```python
from build123d import *

# Parameters (mm, degrees)
SALIENTE_EXTRUIR1_DEPTH = 1.5


with BuildPart() as part:
    # Croquis1 → Saliente-Extruir1 (new, symmetric)
    with BuildSketch(Plane.XY):
        Polygon((484.855720511, 82.973038085), (491.215178715, 82.973038085), (501.205555648, 82.973038085), (501.205555648, 73.173108985), (504.205555648, 73.173108985), (504.205555648, 63.173108985), (501.205555648, 63.173108985), (501.205555648, 45.073108985), (497.205555648, 45.073108985), (497.205555648, 47.573108985), (494.205555648, 47.573108985), (494.205555648, 45.073108985), (493.205555648, 45.073108985), (493.205555648, 42.073108985), (494.205555648, 42.073108985), (494.205555648, 39.573108985), (497.205555648, 39.573108985), (497.205555648, 42.073108985), (501.205555648, 42.073108985), (501.205555648, 38.173108985), (504.205555648, 38.173108985), (504.205555648, 28.173108985), (501.205555648, 28.173108985), (501.205555648, 12.773108985), (494.855720505, 12.773108985), (479.205555648, 12.773108985), (468.814796849, 4.447241951), (463.814796852, 4.447241951), (465.108892077, 9.276871079), (462.2111146, 10.053328214), (464.799305049, 19.712586471), (467.697082526, 18.936129336), (473.790976943, 41.678852916), (477.654680248, 40.643576736), (477.007632636, 38.22876217), (479.905410114, 37.452305035), (480.552457727, 39.867119601), (481.518383553, 39.608300556), (482.294840689, 42.506078034), (481.328914862, 42.764897079), (481.975962475, 45.179711645), (479.078184996, 45.956168781), (478.431137384, 43.541354215), (474.567434078, 44.576630395), (480.661787289, 67.321066215), (477.764009811, 68.097523349), (480.352200261, 77.756781606), (483.249977738, 76.980324471), align=None)
    extrude(amount=SALIENTE_EXTRUIR1_DEPTH, both=True)


solid = part.part
```
Can you work these out from the model? Positions are in its coordinate system, mm. A direction names the side the tool comes from. Coordinates: 2 decimals unless noted, no trailing zeros. Order: outer loops, then holes, each group sorted by start corner. A loop starts at its lowest first (then second) coordinate and runs counter-clockwise, first axis right, second up. Notation, with made-up numbers: (8, 53.25) - (43, 53.25) arc R24 cw to (43, 70.25) - close; hole circle Ø6 at (63, -24). An arc over 180 degrees is marked (long way). Answer in a Markdown table with one row per item.
1. If we mould it in two halves opening along Y, with no side actions, what happens to faces 1 (the flat face through (481.65, 43.96, 0.02)), 2 (the flat face through (493, 82.973, 0)), 3 (the flat face through (504.206, 33, 0))? For each: pulls with the +Y half, pulls with the -Y half, needs draft (parallel to the pull), parting line crosses it, or undercut.
Reply:
| item | result |
|---|---|
| face 1 | undercut |
| face 2 | pulls with the +Y half |
| face 3 | needs draft |
2. Suppose I cut it at C-C (x = 491.5). Please give me the cut outline in (y, z).
Reply:
| item | result |
|---|---|
| outline | (12.77, -1.5) - (82.97, -1.5) - (82.97, 1.5) - (12.77, 1.5) - close |
3. Suppose I cut it at D-D (y = 23). Please give me the cut outline in (x, z).
Reply:
| item | result |
|---|---|
| outline | (468.79, -1.5) - (501.21, -1.5) - (501.21, 1.5) - (468.79, 1.5) - close |
4. If I drill on line 1 along Y through (x, z) = (494, 0.4); line 2 along X through (y, z) = (46, 1.05); line 3 along Y through (x, z) = (488.5, -0.7), over which ranges is the centre line in solid material (lowest first)?
Reply:
| item | result |
|---|---|
| line 1 | y = 12.77 to 42.07, 45.07 to 82.97 |
| line 2 | x = 474.95 to 494.21, 497.21 to 501.21 |
| line 3 | y = 12.77 to 82.97 |
5. Suppose I cut it at B-B (x = 475.5). Please give me the cut outline in (y, z).
Reply:
| item | result |
|---|---|
| outline | (9.8, -1.5) - (41.22, -1.5) - (41.22, 1.5) - (9.8, 1.5) - close; (44.33, -1.5) - (48.06, -1.5) - (48.06, 1.5) - (44.33, 1.5) - close |
6. For faces 4 (the flat face through (479.233, 67.704, 0.021)), 5 (the flat face through (494.206, 41, 0)), 6 (the flat face through (466.23, 19.33, 0.02)), 7 (the flat face through (493.206, 44, 0)), which set-ups out of +Z, -Z, +X, -X, +Y, -Y let a thin tool reach every point of the face, with its end or its side?
Reply:
| item | result |
|---|---|
| face 4 | +Z, -Z, -X |
| face 5 | +Z, -Z |
| face 6 | +Z, -Z, +Y |
| face 7 | +Z, -Z, +X |
7. Suppose I cut it at A-A (x = 498). Please give me the cut outline in (y, z), and give its area (3 significant figures).
Reply:
| item | result |
|---|---|
| outline | (12.77, -1.5) - (42.07, -1.5) - (42.07, 1.5) - (12.77, 1.5) - close; (45.07, -1.5) - (82.97, -1.5) - (82.97, 1.5) - (45.07, 1.5) - close |
| area | 202 mm^2 |
8. For pin 1 (1.5 mm diameter, centred on x = 496, z = 0.5, fed in from -Y); pin 2 (0.9 mm diameter, centred on y = 79.5, z = -0.5, fed in from +X); pin 3 (0.9 mm diameter, centred on x = 502.5, z = 0.5, fed in from +Y), each with a flat end and sliding along its axis, tell me the tip position at first contact or that it passes through.
Reply:
| item | result |
|---|---|
| pin 1 | stops at y = 12.77 |
| pin 2 | stops at x = 501.21 |
| pin 3 | stops at y = 73.17 |
